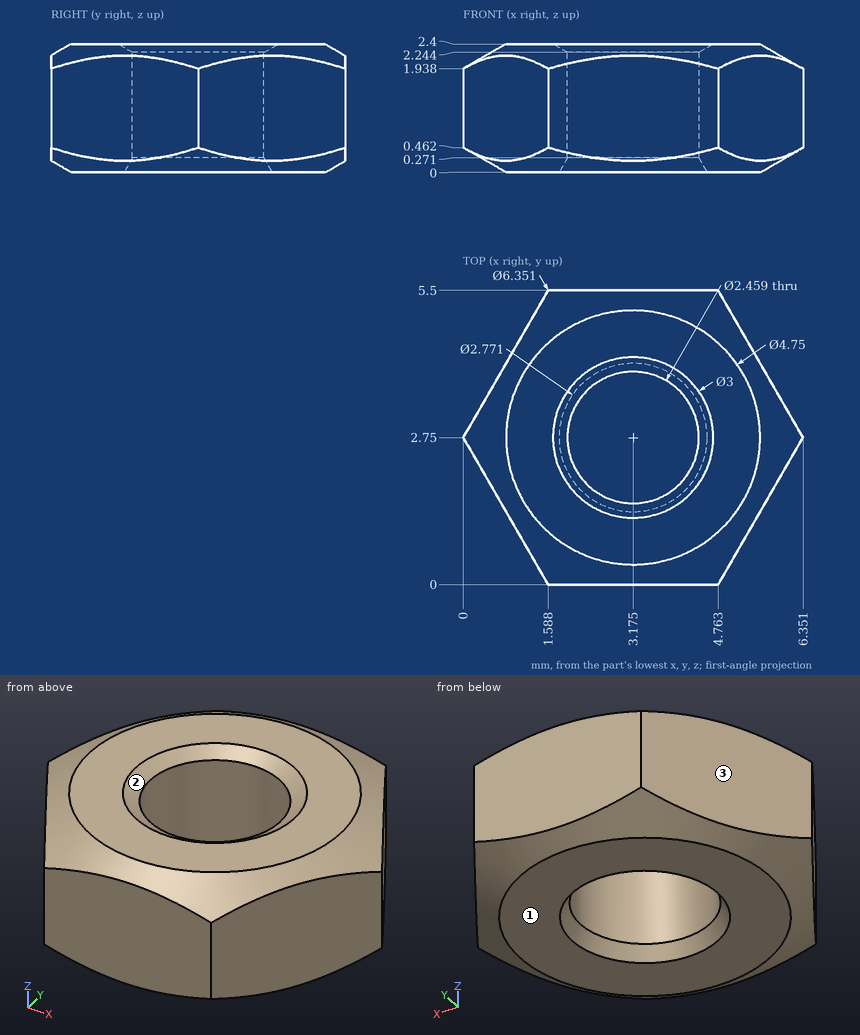
Input: dimensioned drawing with shaded views. Units: mm. Origin: part minimum x, y, z. Give positions to 0.01 mm unless a question says otherwise; leave off trailing zeros.
1. Draft query along X for the marked faces 1, 2 and 3. Return one class per face: released by +X, released by -X, zero draft, split by the parting line, or undercut.
2. Pin query (flat end, axial travel): P1, Ø2, axis at x = 3.18, y = 2.75, coming from the -Z side; P2, Ø1, axis at y = 4.5, z = 2, coming from the +X side. Return the tip coordinate at first contact, or that it passes through.
3. Line query: probe 1 along Y at (x, z) = (2.75, 2.05) (1 decimal); probe 2 along Y at (x, z) = (4, 2.2) (1 decimal); probe 3 along X at (y, z) = (5.1, 0.6) (1 decimal). Output: solid intervals per line, ascending.
Computed:
1. face 1: zero draft
1. face 2: undercut
1. face 3: released by -X
2. P1: passes through
2. P2: stops at x = 5.63
3. probe 1: y = 0 to 1.6, 3.9 to 5.5
3. probe 2: y = 0.2 to 1.8, 3.7 to 5.3
3. probe 3: x = 1.4 to 5
